from build123d import *

# Parameters (mm, degrees)
F0_W     = 150
F0_H     = 100
F1_DEPTH = 15
F2_W     = 50
F2_H     = 80
F3_DEPTH = 24.4
F5_R     = 2
F6_DEPTH = 64.2


with BuildPart() as f1:
    # F0 (on Top) → F1 (new body)
    with BuildSketch(Plane.XY):
        Rectangle(F0_W, F0_H)
    extrude(amount=F1_DEPTH)

    # F2 (on face) → F3 (join)
    with BuildSketch(Plane.XY.offset(15)):
        with Locations((-50, 0)):
            Rectangle(F2_W, F2_H)
    extrude(amount=F3_DEPTH)

    # F5 (on face) → F6 (cut)
    with BuildSketch(Plane(origin=(7.2, 0, 7.2), x_dir=(0, -1, 0), z_dir=(-0.707107, 0, -0.707107))):
        with Locations((25.850689, 31.300105)):
            Circle(F5_R)
    extrude(amount=F6_DEPTH, mode=Mode.SUBTRACT)


solid = f1.part
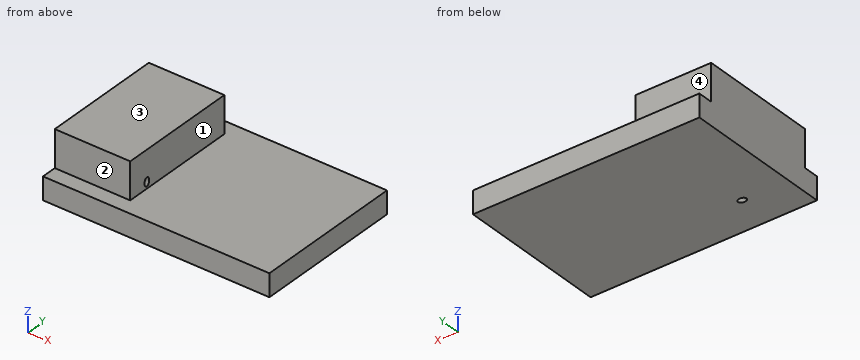
Can you work these out from the model? Positions are in its coordinate system, mm. Face numbers are marked on the shaded views. A direction names the side the tool comes from. Give positions to 0.01 mm unless a question says otherwise; leave off trailing zeros. Loops run counter-clockwise (first coordinate to the right, second up) from the corner with the lowest first, then second, coordinate; pieces in that order, holes last. Notation, with made-up numbers: (-31, 42.5) - (22, 42.5) arc R26 cw to (22, 70.5) - close; hole circle Ø9 at (16.5, -1.5). An arc over 180 degrees is marked (long way). Answer as a JSON object with one key per item and string values.
Q1. Imagine slicing it at C-C on z = 25. Write out the boundary of the cut face in (x, y), plus the area to 3 significant figures.
Geometry says:
{"outline": "(-75, -40) - (-25, -40) - (-25, 40) - (-75, 40) - close", "area": "4,000 mm²"}
Q2. Imagine slicing it at B-B on y = -5. Write out the boundary of the cut face in (x, z).
Geometry says:
{"outline": "(-75, 0) - (75, 0) - (75, 15) - (-25, 15) - (-25, 39.4) - (-75, 39.4) - close"}
Q3. If I drill on L1, parallel to Y at x = -56, z = 37; L2, parallel to X at y = 3, z = 35.5; L3, parallel to Z at x = -22.5, y = -10, over which ranges is the centre line in solid material (lowest first)?
Geometry says:
{"L1": "-40 to 40", "L2": "-75 to -25", "L3": "0 to 15"}
Q4. Imagine slicing it at A-A on x = -59.5. Write out the boundary of the cut face in (y, z), plus the area to 3 significant figures.
Geometry says:
{"outline": "(-50, 0) - (50, 0) - (50, 15) - (40, 15) - (40, 39.4) - (-40, 39.4) - (-40, 15) - (-50, 15) - close", "area": "3,450 mm²"}
Q5. Imagine slicing it at D-D on x = 30. Write out the boundary of the cut face in (y, z).
Geometry says:
{"outline": "(-50, 0) - (50, 0) - (50, 15) - (-50, 15) - close"}
Q6. Will these pins go through, and if not, where does the flat tip stop? P1, Ø19.5, axis at y = 15.5, z = 29.5, coming from the +X side; P2, Ø4, axis at x = -9, y = -33.5, coming from the +Z side; P3, Ø10, axis at x = -58, z = 28.5, coming from the -Y side.
Geometry says:
{"P1": "x = -25", "P2": "z = 15", "P3": "y = -40"}
Q7. Which directions (+Z, -Z, +X, -X, +Y, -Y) give clear straight access to the entire face, cutting with the end or side of a thin tool? Please do the marked faces 1, 2, 3 and 4.
Geometry says:
{"face 1": "+Z, +X, +Y, -Y", "face 2": "+Z, +X, -X, -Y", "face 3": "+Z, +X, -X, +Y, -Y", "face 4": "+Z, +X, -X, +Y"}
